Source: three-view drawing plus pictorial views. Frame: mm from the lowest corner of the part. Round coordinates to 2 decimals unless told otherwise and drop trailing zeros. Order: outer loops, then holes, each group sorted by start corner. A loop starts at its lowest first (then second) coordinate and runs counter-clockwise, first axis right, second up. Notation, with made-up numbers: (14, -12) -> (22, -12) arc R27 ccw to (22, 20) -> close; hole circle Ø11 at (-0.75, 75.25). An arc over 180 degrees is marked (long way). Answer as CSV lines item,"result".
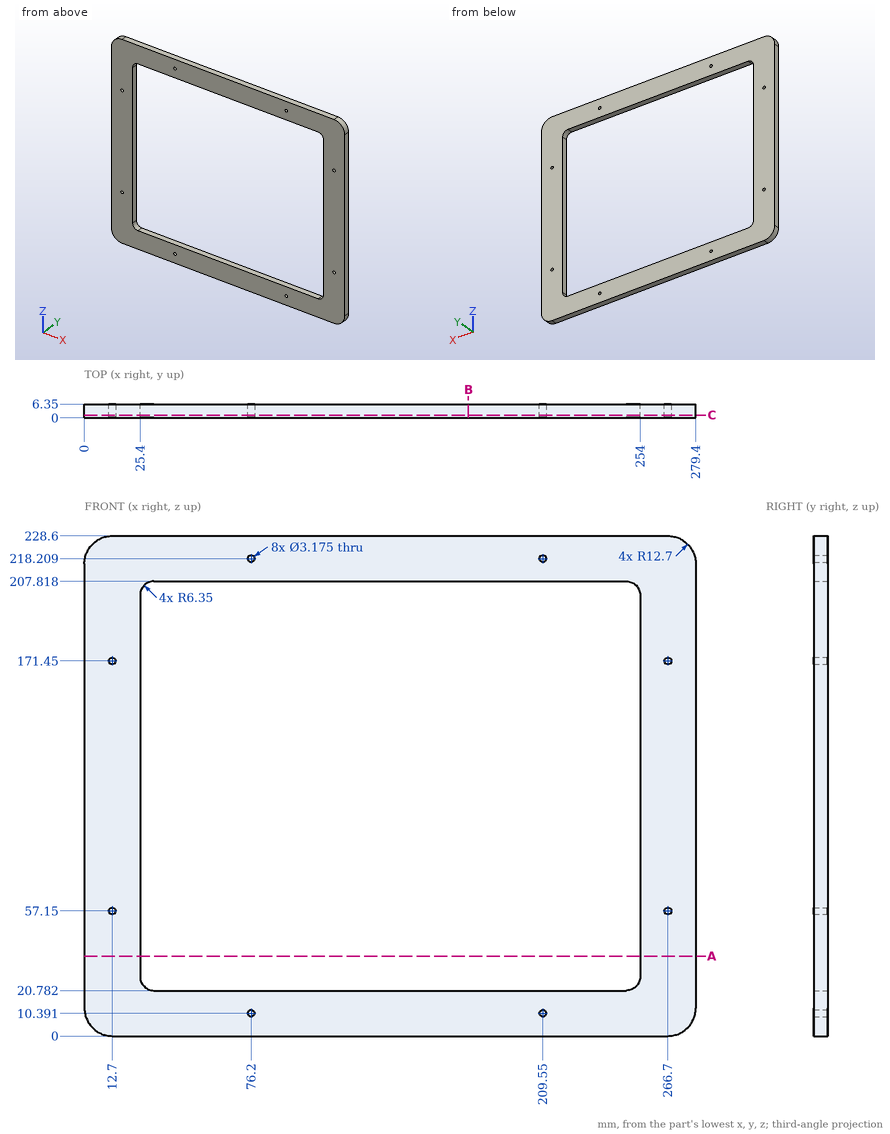
1. Line query: L1, parallel to Z at x = 76.2, y = 1.5; L2, parallel to Z at x = 266.7, y = 1.5; L3, parallel to X at y = 4.25, z = 57.15. Output: solid intervals per line, ascending. Write a range as [from, to].
Results below:
L1,"[0, 8.8], [11.98, 20.78], [207.82, 216.62], [219.8, 228.6]"
L2,"[0, 55.56], [58.74, 169.86], [173.04, 228.6]"
L3,"[0, 11.11], [14.29, 25.4], [254, 265.11], [268.29, 279.4]"
2. Section query A-A on z = 36.5. Return loops of the section in (x, y).
Results below:
outline,"(0, 0) -> (25.4, 0) -> (25.4, 6.35) -> (0, 6.35) -> close; (254, 0) -> (279.4, 0) -> (279.4, 6.35) -> (254, 6.35) -> close"
3. Section query C-C on y = 1.25. Give the number of separate pieces and of enclosed holes in the cut face, and give its area (3 significant figures).
Results below:
separate pieces,"1"
enclosed holes,"9"
area,"20,900 mm2"
4. Section query B-B on x = 175.5. Return loops of the section in (y, z).
Results below:
outline,"(0, 0) -> (6.35, 0) -> (6.35, 20.78) -> (0, 20.78) -> close; (0, 207.82) -> (6.35, 207.82) -> (6.35, 228.6) -> (0, 228.6) -> close"
